Autodesk Inventor part; units mm, degrees
ref_plane "Plano inicial" through (0, 0, 0) normal (0, 0, 1) x (1, 0, 0)
ref_plane "Plano final" through (0, 0, 450) normal (0, 0, 1) x (1, 0, 0)
ref_plane "Plano de trabalho6" through (155, 0, 450) normal (0, 0, 1) x (1, 0, 0)
ref_plane "Plano inicial" through (0, 0, 0) normal (0, 0, 1) x (1, 0, 0)
ref_plane "Plano final" through (0, 0, 450) normal (0, 0, 1) x (1, 0, 0)
sketch "Esboço" plane through (0, 0, 0) normal (0, 0, 1) x (1, 0, 0)
  line L0 (-15, -11) -> (-15, 11)
  line L1 (-11, 15) -> (11, 15)
  line L2 (15, 11) -> (15, -11)
  line L3 (11, -15) -> (-11, -15)
  arc A0 (-15, -11) -> (-11, -15) centre (-11, -11) ccw
  arc A1 (15, 11) -> (11, 15) centre (11, 11) ccw
  arc A2 (-11, 15) -> (-15, 11) centre (-11, 11) ccw
  arc A3 (11, -15) -> (15, -11) centre (11, -11) ccw
  arc A4 (-11, 13) -> (-13, 11) centre (-11, 11) ccw
  line L4 (-11, 13) -> (11, 13)
  arc A5 (13, 11) -> (11, 13) centre (11, 11) ccw
  line L5 (13, 11) -> (13, -11)
  arc A6 (11, -13) -> (13, -11) centre (11, -11) ccw
  line L6 (11, -13) -> (-11, -13)
  arc A7 (-13, -11) -> (-11, -13) centre (-11, -11) ccw
  line L7 (-13, -11) -> (-13, 11)
  line L8 (0, 22.1598) -> (0, -22.1598) construction
  line L9 (-22.1598, 0) -> (22.1598, 0) construction
  dimension "d7" = 4
  dimension "d9" = 30
  dimension "d11" = 30
  dimension "d12" = 2
  dimension "d15" = 15
  dimension "d16" = 15
extrude "Corpo" add sketch "Esboço" along normal up to surface (450 mm away) from surface at 0
sketch "Sketch3" plane through (0, 0, 0) normal (0, 0, 1) x (1, 0, 0)
  line L0 (0, 0) -> (10, 0)
ref_plane "Work Plane3" through (0, 0, 0) normal (0, -1, 0) x (1, 0, 0)
sketch "Sketch4" plane through (0, 0, 0) normal (0, -1, 0) x (1, 0, 0)
  line L0 (-2, 0) -> (12, 0)
  line L1 (-2, 450) -> (12, 450)
  dimension "d18" = 450
ref_plane "Plano de trabalho6" through (155, 0, 450) normal (0, 0, 1) x (1, 0, 0)
split "Dividir3" plane through (155, 0, 450) removes the side toward (0, 0, 1)
ref_plane "Plano de trabalho7" through (0, 15, 0) normal (0, -0.7071, -0.7071) x (1, 0, 0)
split "Dividir4" plane through (0, 15, 0) removes the side toward (0, -0.7071, -0.7071)
ref_plane "Plano de trabalho8" through (0, 15, 450) normal (0, -0.7071, 0.7071) x (1, 0, 0)
split "Dividir5" plane through (0, 15, 450) removes the side toward (0, -0.7071, 0.7071)
equation "\"d7\" = G_IR"
equation "\"d9\" = G_W"
equation "\"d11\" = G_H"
equation "\"d12\" = G_T"
equation "\"d15\" = 0.5 * d9"
equation "\"d16\" = 0.5 * d11"
equation "\"d3\" = G_L"
equation "\"G_W\" = 30"
equation "\"G_H\" = 30"
equation "\"G_T\" = 2"
equation "\"G_IR\" = 4"
equation "\"G_L\" = d18"
equation "\"G_OFFSET_START\" = 0"
equation "\"G_OFFSET_END\" = 0"
properties part number "ISO 10799-2 - 30x30x2 - 450" material "Aço, suave"
Geometry check sheet. Reference: the model listing, model coordinates, mm. A direction names the side the tool comes from. Round coordinates to 2 decimals unless told otherwise and drop trailing zeros. Loops run counter-clockwise (first coordinate to the right, second up) from the corner with the lowest first, then second, coordinate; pieces in that order, holes last. Notation, with made-up numbers: (25, 83.25) - (83, 83.25) arc R17 cw to (83, 109.25) - close; hole circle Ø11 at (70.5, 75.5). An arc over 180 degrees is marked (long way). Use a Markdown table: item, result.
Q1. Draft check along X on faces 1 (the flat face through (-15, 0, 222)), 2 (the flat face through (0, -13, 222)), 3 (the flat face through (13, 0, 222)), 4 (the flat face through (-14, 0, 435)). Enter one of: released by +X, released by -X, zero draft, split by the parting line, or undercut.
Solutions:
| item | result |
|---|---|
| face 1 | released by -X |
| face 2 | undercut |
| face 3 | undercut |
| face 4 | zero draft |
Q2. Access from +Z, -Z, +X, -X, +Y, -Y to the whole of each face (thin tool, end or side, straight path). Record for faces 5 (the flat face through (0, 13, 222)), 6 (the flat face through (0, 15, 222)).
Solutions:
| item | result |
|---|---|
| face 5 | +Z, -Z |
| face 6 | +Z, -Z, +X, -X, +Y |
Q3. Material ranges on line 1 (Y direction, x = -1.5, z = 41); line 2 (Y direction, x = 11.5, z = 192), recorded low to high.
Solutions:
| item | result |
|---|---|
| line 1 | y = -15 to -13, 13 to 15 |
| line 2 | y = -14.97 to -12.94, 12.94 to 14.97 |
Q4. Cross-section at A-A on y = -1. Record the cut outline in (x, z), plus the area to 3 significant figures.
Solutions:
| item | result |
|---|---|
| outline | (-15, 16) - (-13, 16) - (-13, 434) - (-15, 434) - close; (13, 16) - (15, 16) - (15, 434) - (13, 434) - close |
| area | 1,670 mm2 |
Q5. Cross-section at C-C on z = 141. Record the cut outline in (x, y).
Solutions:
| item | result |
|---|---|
| outline | (-15, -11) arc R4 ccw to (-11, -15) - (11, -15) arc R4 ccw to (15, -11) - (15, 11) arc R4 ccw to (11, 15) - (-11, 15) arc R4 ccw to (-15, 11) - close; hole (-13, -11) arc R2 ccw to (-11, -13) - (11, -13) arc R2 ccw to (13, -11) - (13, 11) arc R2 ccw to (11, 13) - (-11, 13) arc R2 ccw to (-13, 11) - close |
Q6. Cross-section at B-B on x = -0.5. Record the cut outline in (y, z), plus the area to 3 significant figures.
Solutions:
| item | result |
|---|---|
| outline | (-15, 30) - (-13, 28) - (-13, 422) - (-15, 420) - close; (13, 2) - (15, 0) - (15, 450) - (13, 448) - close |
| area | 1,680 mm2 |
